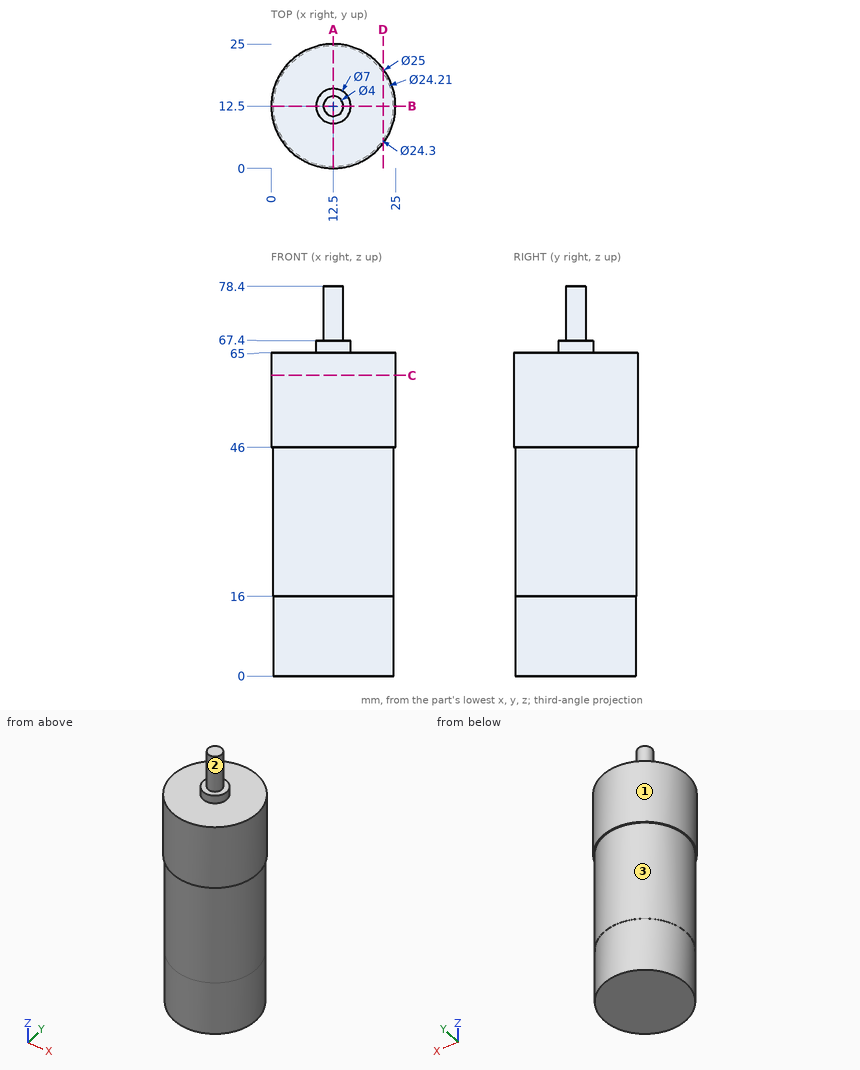
Verification items for this drawing (mm, ordinates from the low corner). A direction names the side the tool comes from. Coordinates: 2 decimals unless noted, no trailing zeros. Order: outer loops, then holes, each group sorted by start corner. A loop starts at its lowest first (then second) coordinate and runs counter-clockwise, first axis right, second up. Notation, with made-up numbers: M 71.5,-28 L 85.5,-28 A16 ccw 85.5,-14 Z; hole C 64.25,2 d10. An arc over 180 degrees is marked long. Answer as a JSON object with one key per item and string values.
Q1. Scan lines: line 1 (Z direction, x = 9.25, y = 2.5); line 2 (Y direction, x = 12.25, z = 13.5); line 3 (X direction, y = 4.5, z = 5.5). Record each from-to range of solid material in increasing order.
Results are:
{"line 1": "z = 0 to 65", "line 2": "y = 0.4 to 24.6", "line 3": "x = 3.42 to 21.58"}
Q2. Cross-section at D-D on x = 22.5. Record the cut outline in (y, z).
Results are:
{"outline": "M 5,46 L 5.6,46 L 5.6,16 L 5.68,16 L 5.68,0 L 19.32,0 L 19.32,16 L 19.4,16 L 19.4,46 L 20,46 L 20,65 L 5,65 Z"}
Q3. Cross-section at A-A on x = 12.5. Record the cut outline in (y, z) (3 decimals), and give its area (3 significant figures).
Results are:
{"outline": "M 0,46 L 0.35,46 L 0.35,16 L 0.395,16 L 0.395,0 L 24.605,0 L 24.605,16 L 24.65,16 L 24.65,46 L 25,46 L 25,65 L 16,65 L 16,67.4 L 14.5,67.4 L 14.5,78.4 L 10.5,78.4 L 10.5,67.4 L 9,67.4 L 9,65 L 0,65 Z", "area": "1,650 mm²"}
Q4. Tool access check on the marked faces 1, 2 and 3. Record the directions out of +Z, -Z, +X, -X, +Y, -Y that give a thin tool (end or side, any length) a straight path to the whole face; none if there is none.
Results are:
{"face 1": "+Z, -Z", "face 2": "+Z", "face 3": "-Z"}
Q5. Cross-section at C-C on z = 60.5. Record the cut outline in (x, y).
Results are:
{"outline": "C 12.5,12.5 d25"}
Q6. Depth check by flat-ended pin: pin 1 Ø8 at (x, y) = (16, 5.5) entering from +Z; pin 2 Ø4 at (x, y) = (15, 8) entering from +Z; pin 3 Ø8 at (x, z) = (12, 17) entering from -Y. Enter the tip coordinate at first touch or a pass-through.
Results are:
{"pin 1": "stops at z = 65", "pin 2": "stops at z = 67.4", "pin 3": "stops at y = 0.35"}
